Here's the drawing with two shaded views (mm, measured from the low corner). I have some questions. A direction names the side the tool comes from. Give positions to 0.01 mm unless a question says otherwise; leave off trailing zeros. Write each loop counter-clockwise with the first axis right and the second up, starting at its lowest first coordinate (ties: lowest second). Pieces come first, ordered by that corner, then holes. Notation, with made-up numbers: (-10.75, 26) -> (39.25, 26) arc R20 ccw to (39.25, 54) -> close; hole circle Ø5 at (9.25, 71.25). An arc over 180 degrees is marked (long way). One line per item, written item: value.
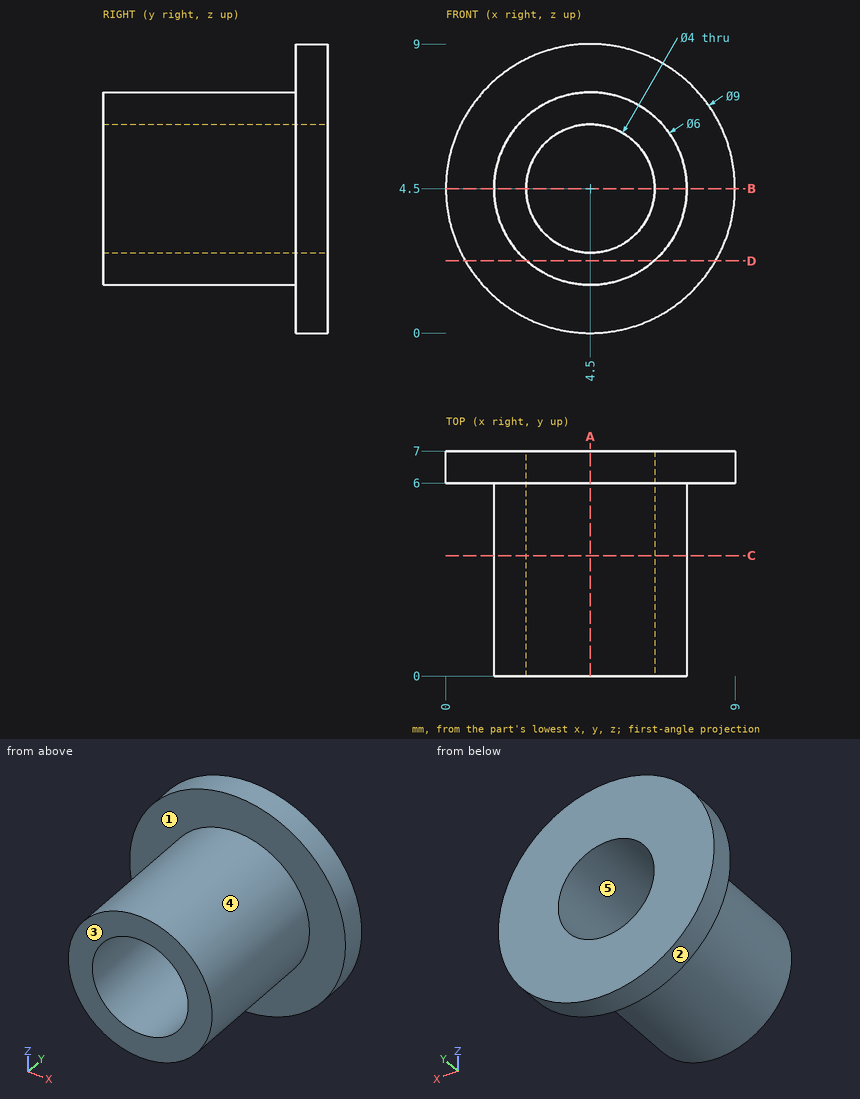
1) If we section it at D-D (z = 2.25): Write out the boundary of the cut face in (x, y).
Answer list:
outline: (0.6, 6) -> (2.52, 6) -> (2.52, 0) -> (6.48, 0) -> (6.48, 6) -> (8.4, 6) -> (8.4, 7) -> (0.6, 7) -> close
2) Will these pins go through, and if not, where does the flat tip stop? pin 1 (1.5 mm diameter, centred on x = 6, y = 1, fed in from +Z); pin 2 (1.5 mm diameter, centred on y = 3, z = 8, fed in from -X); pin 3 (2 mm diameter, centred on y = 3, z = 6, fed in from +X).
Answer list:
pin 1: stops at z = 7.4
pin 2: stops at x = 3.3
pin 3: stops at x = 7.46
3) For the marked faces 1 and 2, which set-ups out of +Z, -Z, +X, -X, +Y, -Y let a thin tool reach every point of the face, with its end or its side?
Answer list:
face 1: -Y
face 2: +Y, -Y
4) If we section it at A-A (x = 4.5): Write out the boundary of the cut face in (y, z), and give its area (3 significant figures).
Answer list:
outline: (0, 1.5) -> (6, 1.5) -> (6, 0) -> (7, 0) -> (7, 2.5) -> (0, 2.5) -> close; (0, 6.5) -> (7, 6.5) -> (7, 9) -> (6, 9) -> (6, 7.5) -> (0, 7.5) -> close
area: 17.0 mm^2
5) We'd pull the mould along Z, two halves only. Please class the marked faces 3, 4 and 5: released by +Z, released by -Z, zero draft, split by the parting line, or undercut.
Answer list:
face 3: zero draft
face 4: split by the parting line
face 5: undercut
6) If we section it at B-B (z = 4.5): Write out the boundary of the cut face in (x, y), and give its area (3 significant figures).
Answer list:
outline: (0, 6) -> (1.5, 6) -> (1.5, 0) -> (2.5, 0) -> (2.5, 7) -> (0, 7) -> close; (6.5, 0) -> (7.5, 0) -> (7.5, 6) -> (9, 6) -> (9, 7) -> (6.5, 7) -> close
area: 17.0 mm^2
7) I need wall thicknesses on L1, parallel to Z at x = 4.5, y = 4.5; L2, parallel to Y at x = 8.75, z = 5.75. Which ranges of each line are inside material? Lowest first, please.
Answer list:
L1: z = 1.5 to 2.5, 6.5 to 7.5
L2: y = 6 to 7
8) If we section it at C-C (y = 3.75): Write out the boundary of the cut face in (x, z), and give its area (3 significant figures).
Answer list:
outline: circle Ø6 at (4.5, 4.5); hole circle Ø4 at (4.5, 4.5)
area: 15.7 mm^2
